Design review of the part built by this model. Coordinates are the model's own, in mm. Face numbers are marked on the shaded views. A direction names the side the tool comes from. Give positions to 0.01 mm unless a question says otherwise; leave off trailing zeros. Loops run counter-clockwise (first coordinate to the right, second up) from the corner with the lowest first, then second, coordinate; pieces in that order, holes last. Notation, with made-up numbers: (88, 88.25) -> (126, 88.25) arc R24 cw to (126, 123.25) -> close; hole circle Ø8 at (19, 70). An arc over 180 degrees is marked (long way). Answer in a Markdown table with one row per item. Add a question column.
(1) Draft analysis for pull direction X (two halves, no side actions). For the marked faces 1, 2, 3 and 4, state which applies: +X half, -X half, draft (parallel to the pull), parting line (faces both ways), or undercut.
(2) Consider section B-B on x = -27. Write out the cut boundary in (y, z), then the cut area to 3 significant figures.
(3) For the marked faces 5, 6, 7 and 8, list the 3-axis set-ups (+Z, -Z, +X, -X, +Y, -Y) from which the entire face can be reached by the end or side of a thin tool; tool diameter is ignored.
(4) For line 1 (Y direction, x = 2, z = 30.45); line 2 (X direction, y = 40, z = 30.3); line 3 (Y direction, x = -13.5, z = 38.5), list the stretches that pass through material, from the lowest coordinate up.
(5) Consider section A-A on y = 5. Write out the cut boundary in (x, z).
(6) Consider section C-C on z = 34.75. Write out the cut boundary in (x, y).
(7) Consider section D-D on y = 28. Write out the cut boundary in (x, z), then the cut area to 3 significant figures.
(8) For pin 1 (1.3 mm diameter, centred on x = -30, y = 10.5, fed in from +Z); pin 2 (3 mm diameter, centred on x = 3, y = 5, fed in from +Z); pin 3 (3 mm diameter, centred on y = 23, z = 38.5, fed in from +X); pin 4 (2.5 mm diameter, centred on x = -29.5, y = 10.5, fed in from +Z), all flat-tipped, find the tip position at first contact; note any pin that passes through.
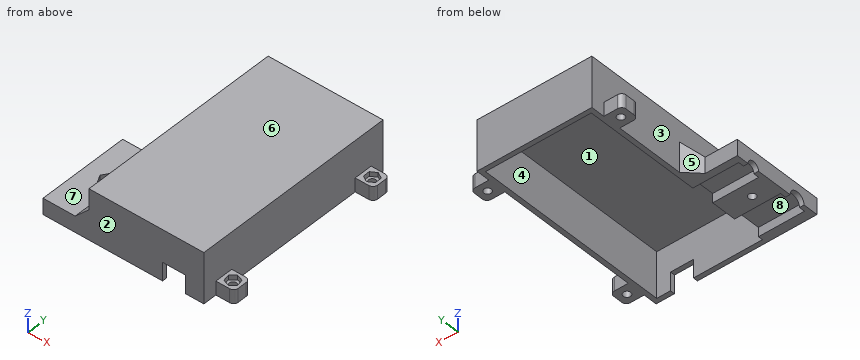
from build123d import *

# Parameters (mm, degrees)
SKETCH_W        = 25
SKETCH_H        = 45
PAD_DEPTH       = 11
SKETCH001_W     = 20
SKETCH001_H     = 3.5
PAD001_DEPTH    = 10
SKETCH002_R     = 1.75
SKETCH002_R_2   = 1.311362
POCKET_DEPTH    = 12
SKETCH003_W     = 11
SKETCH003_H     = 5
SKETCH003_H_2   = 6
POCKET001_DEPTH = 2
SKETCH005_W     = 23
SKETCH005_H     = 43
POCKET002_DEPTH = 10
CHAMFER_SIZE    = 3
CHAMFER001_SIZE = 3
SKETCH006_W     = 5
SKETCH006_H     = 4
POCKET003_DEPTH = 1
SKETCH007_R     = 0.8
POCKET004_DEPTH = 5
POCKET005_DEPTH = 2
SKETCH009_W     = 4
SKETCH009_H     = 4
PAD002_DEPTH    = 3
SKETCH010_R     = 0.8
POCKET006_DEPTH = 5
POCKET007_DEPTH = 1
SKETCH012_R     = 0.8
POCKET008_DEPTH = 5
POCKET009_DEPTH = 1
SKETCH014_R     = 0.8
POCKET010_DEPTH = 5
POCKET011_DEPTH = 1
FILLET_R        = 1
FILLET001_R     = 1
FILLET002_R     = 1
FILLET003_R     = 1
FILLET004_R     = 1
FILLET005_R     = 1


with BuildPart() as pad:
    # Sketch → Pad (new body)
    with BuildSketch(Plane.XY):
        with Locations((-12.5, 22.5)):
            Rectangle(SKETCH_W, SKETCH_H)
    extrude(amount=PAD_DEPTH)


with BuildPart() as pad001:
    # Pad001 base: copy of Pad
    add(pad.part)

    # Sketch001 (on Face2 of Pad) → Pad001 (new body)
    with BuildSketch(Plane(origin=(-25, 0, 0), x_dir=(0, -1, 0), z_dir=(-1, 0, 0))):
        with Locations((-10, 9.25)):
            Rectangle(SKETCH001_W, SKETCH001_H)
    extrude(amount=PAD001_DEPTH)


with BuildPart() as fillet005:
    # Fusion base: copy of Pad
    add(pad.part)

    # Fusion: union Pad001
    add(pad001.part)

    # Sketch002 (on Face1 of Fusion) → Pocket (cut)
    with BuildSketch(Plane(origin=(-35, 0, 0), x_dir=(0, -1, 0), z_dir=(-1, 0, 0))):
        with Locations((-5, 11)):
            Circle(SKETCH002_R)
        with Locations((-16, 11)):
            Circle(SKETCH002_R_2)
    extrude(amount=-POCKET_DEPTH, mode=Mode.SUBTRACT)

    # Sketch003 (on Face6 of Pocket) → Pocket001 (cut)
    with BuildSketch(Plane.XY.offset(11)):
        with Locations((-28.5, 16)):
            Rectangle(SKETCH003_W, SKETCH003_H)
        with Locations((-28.5, 5)):
            Rectangle(SKETCH003_W, SKETCH003_H_2)
    extrude(amount=-POCKET001_DEPTH, mode=Mode.SUBTRACT)

    # Sketch005 (on Face10 of Pocket001) → Pocket002 (cut)
    with BuildSketch(Plane.XY.offset(11)):
        with Locations((-12.5, 22.5)):
            Rectangle(SKETCH005_W, SKETCH005_H)
    extrude(amount=-POCKET002_DEPTH, mode=Mode.SUBTRACT)

    # Chamfer
    chamfer_edges = [fillet005.edges().sort_by_distance(p)[0] for p in [
        (-25, 10, 7.5),
    ]]
    chamfer(chamfer_edges, length=CHAMFER_SIZE)

    # Chamfer001
    chamfer001_edges = [fillet005.edges().sort_by_distance(p)[0] for p in [
        (-25, 20, 9.25),
        (-25, 20, 6),
    ]]
    chamfer(chamfer001_edges, length=CHAMFER001_SIZE)

    # Sketch006 (on Face12 of Chamfer001) → Pocket003 (cut)
    with BuildSketch(Plane.XZ):
        with Locations((-6.5, 9)):
            Rectangle(SKETCH006_W, SKETCH006_H)
    extrude(amount=-POCKET003_DEPTH, mode=Mode.SUBTRACT)

    # Sketch007 (on Face16 of Pocket003) → Pocket004 (cut)
    with BuildSketch(Plane.XY.offset(11)):
        with Locations((-30, 10.5)):
            Circle(SKETCH007_R)
    extrude(amount=-POCKET004_DEPTH, mode=Mode.SUBTRACT)

    # Sketch008 (on Face3 of Pocket004) → Pocket005 (cut)
    with BuildSketch(Plane(origin=(0, 0, 7.5), x_dir=(1, 0, 0), z_dir=(0, 0, -1))):
        Polygon((-29.047812, -12), (-28.224868, -10.425381), (-29.177056, -8.925381), (-30.952188, -9), (-31.775132, -10.574619), (-30.822944, -12.074619), align=None)
    extrude(amount=-POCKET005_DEPTH, mode=Mode.SUBTRACT)

    # Sketch009 (on Face15 of Pocket005) → Pad002 (new body)
    with BuildSketch(Plane.XY.offset(11)):
        with Locations((-27, 40)):
            Rectangle(SKETCH009_W, SKETCH009_H)
        with Locations((2, 40)):
            Rectangle(SKETCH009_W, SKETCH009_H)
        with Locations((2, 5)):
            Rectangle(SKETCH009_W, SKETCH009_H)
    extrude(amount=-PAD002_DEPTH)

    # Sketch010 (on Face33 of Pad002) → Pocket006 (cut)
    with BuildSketch(Plane.XY.offset(11)):
        with Locations((-27, 40)):
            Circle(SKETCH010_R)
    extrude(amount=-POCKET006_DEPTH, mode=Mode.SUBTRACT)

    # Sketch011 (on Face20 of Pocket006) → Pocket007 (cut)
    with BuildSketch(Plane(origin=(0, 0, 8), x_dir=(1, 0, 0), z_dir=(0, 0, -1))):
        Polygon((-25.520394, -40.24651), (-26.046714, -38.841879), (-27.526319, -38.595369), (-28.479606, -39.75349), (-27.953286, -41.158121), (-26.473681, -41.404631), align=None)
    extrude(amount=-POCKET007_DEPTH, mode=Mode.SUBTRACT)

    # Sketch012 (on Face37 of Pocket007) → Pocket008 (cut)
    with BuildSketch(Plane.XY.offset(11)):
        with Locations((2, 40)):
            Circle(SKETCH012_R)
    extrude(amount=-POCKET008_DEPTH, mode=Mode.SUBTRACT)

    # Sketch013 (on Face59 of Pocket008) → Pocket009 (cut)
    with BuildSketch(Plane(origin=(0, 0, 8), x_dir=(1, 0, 0), z_dir=(0, 0, -1))):
        Polygon((3.289533, -40.766227), (3.308339, -39.266345), (2.018806, -38.500118), (0.710467, -39.233773), (0.691661, -40.733655), (1.981194, -41.499882), align=None)
    extrude(amount=-POCKET009_DEPTH, mode=Mode.SUBTRACT)

    # Sketch014 (on Face40 of Pocket009) → Pocket010 (cut)
    with BuildSketch(Plane.XY.offset(11)):
        with Locations((2, 5)):
            Circle(SKETCH014_R)
    extrude(amount=-POCKET010_DEPTH, mode=Mode.SUBTRACT)

    # Sketch015 (on Face56 of Pocket010) → Pocket011 (cut)
    with BuildSketch(Plane(origin=(0, 0, 8), x_dir=(1, 0, 0), z_dir=(0, 0, -1))):
        Polygon((3.133484, -5.982453), (3.417571, -4.5096), (2.284087, -3.527147), (0.866516, -4.017547), (0.582429, -5.4904), (1.715913, -6.472853), align=None)
    extrude(amount=-POCKET011_DEPTH, mode=Mode.SUBTRACT)

    # Fillet
    fillet_edges = [fillet005.edges().sort_by_distance(p)[0] for p in [
        (-29, 38, 9.5),
    ]]
    fillet(fillet_edges, radius=FILLET_R)

    # Fillet001
    fillet001_edges = [fillet005.edges().sort_by_distance(p)[0] for p in [
        (-29, 42, 9.5),
    ]]
    fillet(fillet001_edges, radius=FILLET001_R)

    # Fillet002
    fillet002_edges = [fillet005.edges().sort_by_distance(p)[0] for p in [
        (4, 42, 9.5),
    ]]
    fillet(fillet002_edges, radius=FILLET002_R)

    # Fillet003
    fillet003_edges = [fillet005.edges().sort_by_distance(p)[0] for p in [
        (4, 38, 9.5),
    ]]
    fillet(fillet003_edges, radius=FILLET003_R)

    # Fillet004
    fillet004_edges = [fillet005.edges().sort_by_distance(p)[0] for p in [
        (4, 7, 9.5),
    ]]
    fillet(fillet004_edges, radius=FILLET004_R)

    # Fillet005
    fillet005_edges = [fillet005.edges().sort_by_distance(p)[0] for p in [
        (4, 3, 9.5),
    ]]
    fillet(fillet005_edges, radius=FILLET005_R)


with BuildPart() as part_mirroring:
    # Part__Mirroring: instance of Fillet005
    add(fillet005.part.mirror(Plane(origin=(0, 0, 20), x_dir=(0, 1, 0), z_dir=(0, 0, 1))))


solid = part_mirroring.part
Values follow:
| question | item | result |
|---|---|---|
| 1 | face 1 | undercut |
| 1 | face 2 | draft |
| 1 | face 3 | -X half |
| 1 | face 4 | undercut |
| 2 | outline | (0, 29) -> (2, 29) -> (2, 31) -> (8, 31) -> (8, 29) -> (13.5, 29) -> (13.5, 31) -> (18.5, 31) -> (18.5, 29) -> (21, 29) -> (21, 33.5) -> (0, 33.5) -> close; (38, 29) -> (39.2, 29) -> (39.2, 31) -> (38.68, 31) -> (38.68, 32) -> (38, 32) -> close; (40.8, 29) -> (42, 29) -> (42, 32) -> (41.32, 32) -> (41.32, 31) -> (40.8, 31) -> close |
| 2 | area | 78.7 mm2 |
| 3 | face 5 | +Z, -Z, -X |
| 3 | face 6 | +Z, +X, -X, +Y, -Y |
| 3 | face 7 | +Z, -X, +Y, -Y |
| 3 | face 8 | -Z |
| 4 | line 1 | 3 to 4.2, 5.8 to 7, 38 to 39.2, 40.8 to 42 |
| 4 | line 2 | -29 to -27.8, -26.2 to -24, -1 to 1.2, 2.8 to 4 |
| 4 | line 3 | 0 to 1, 44 to 45 |
| 5 | outline | (-35, 30.75) -> (-34, 30.75) -> (-34, 31) -> (-24, 31) -> (-24, 39) -> (-1, 39) -> (-1, 29) -> (1.2, 29) -> (1.2, 31) -> (0.68, 31) -> (0.68, 32) -> (0, 32) -> (0, 40) -> (-25, 40) -> (-25, 35.5) -> (-28, 32.5) -> (-35, 32.5) -> close; (2.8, 29) -> (4, 29) -> (4, 32) -> (3.32, 32) -> (3.32, 31) -> (2.8, 31) -> close |
| 6 | outline | (-25.75, 0) -> (0, 0) -> (0, 45) -> (-25, 45) -> (-25, 23) -> (-25.75, 22.25) -> close; hole (-24, 1) -> (-1, 1) -> (-1, 44) -> (-24, 44) -> close |
| 7 | outline | (-25, 29) -> (-24, 29) -> (-24, 39) -> (-1, 39) -> (-1, 29) -> (0, 29) -> (0, 40) -> (-25, 40) -> close |
| 7 | area | 45.0 mm2 |
| 8 | pin 1 | through |
| 8 | pin 2 | z = 32 |
| 8 | pin 3 | x = 0 |
| 8 | pin 4 | z = 32.5 |
